Here's the drawing with two shaded views (mm, measured from the low corner). I have some questions. Round coordinates to 2 decimals unless told otherwise and drop trailing zeros. Loops run counter-clockwise (first coordinate to the right, second up) from the corner with the lowest first, then second, coordinate; pieces in that order, holes last.
(1) If I drill on line 1 along X through (y, z) = (155, 2.3) (1 decimal); line 2 along Y through (x, z) = (42.5, 2.9) (1 decimal); line 3 along X through (y, z) = (148.5, 1.7) (1 decimal), over which ranges is the centre line in solid material (lowest first)?
(2) I want a section at D-D on y = 15. Write out the boundary of the cut face in (x, z) (1 decimal).
(3) Will these pins go through, and if not, where does the flat tip stop? pin 1 Ø5 at (x, y) = (113, 58.5) entering from +Z; pin 2 Ø1.5 at (x, z) = (103, 1) entering from -Y; pin 3 Ø1.5 at (y, z) = (97, 1) entering from -X.
(4) I want a section at C-C on z = 0.9. Write out the boundary of the cut face in (x, y), plus the area to 3 significant figures.
(5) I want a section at A-A on x = 95. Write out the boundary of the cut face in (y, z), plus the area to 3 significant figures.
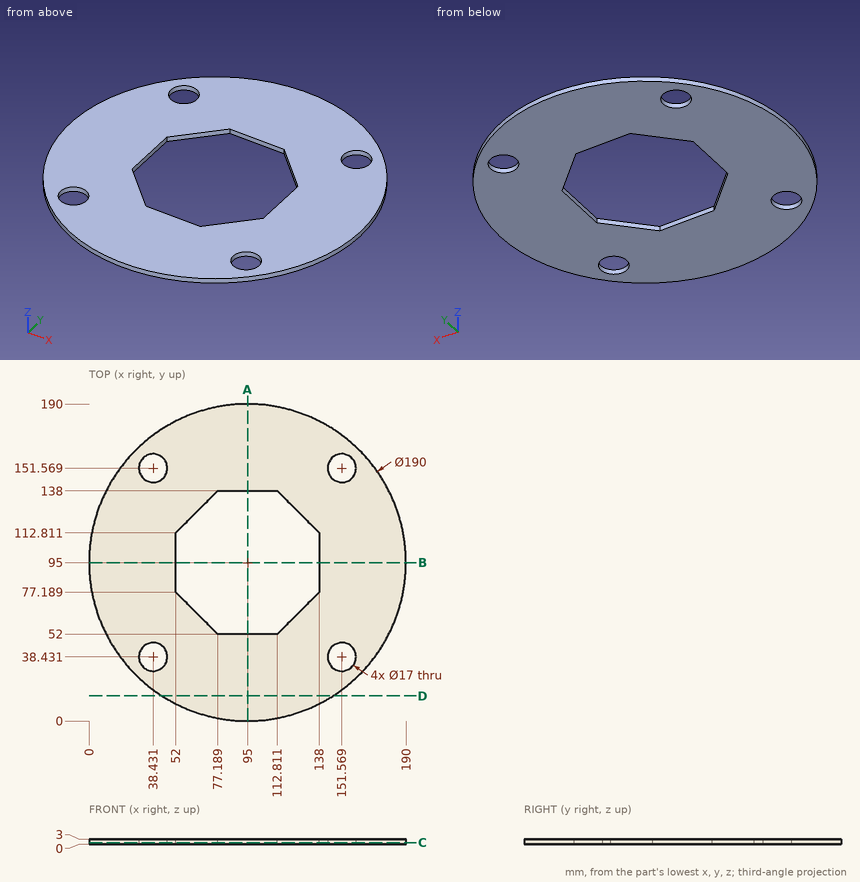
Filled sheet:
1. line 1: x = 21.3 to 30.7, 46.2 to 143.8, 159.3 to 168.7
1. line 2: y = 15.8 to 31, 45.9 to 144.1, 159 to 174.2
1. line 3: x = 16.5 to 30.5, 46.4 to 143.6, 159.5 to 173.5
2. outline: (43.8, 0) - (146.2, 0) - (146.2, 3) - (43.8, 3) - close
3. pin 1: passes through
3. pin 2: stops at y = 0.28
3. pin 3: stops at x = 0.01
4. outline: circle Ø190 at (95, 95); hole circle Ø17 at (38.43, 38.43); hole circle Ø17 at (38.43, 151.57); hole (52, 77.19) - (77.19, 52) - (112.81, 52) - (138, 77.19) - (138, 112.81) - (112.81, 138) - (77.19, 138) - (52, 112.81) - close; hole circle Ø17 at (151.57, 38.43); hole circle Ø17 at (151.57, 151.57)
4. area: 21,300 mm2
5. outline: (0, 0) - (52, 0) - (52, 3) - (0, 3) - close; (138, 0) - (190, 0) - (190, 3) - (138, 3) - close
5. area: 312 mm2
